The listing builds one solid part. Answer for the finished solid, in the listing's coordinates (mm). Coordinates: 2 decimals unless noted, no trailing zeros. Write each loop counter-clockwise with the first axis right and the second up, starting at its lowest first coordinate (ties: lowest second). Pieces come first, ordered by that corner, then holes. Notation, with made-up numbers: M 10.25,34.25 L 67.25,34.25 A23 ccw 67.25,45.25 Z; hole C 75,-27.75 d2. An arc over 180 degrees is marked long. Answer as a JSON object with one key per item and string values. Group by question number.
from build123d import *

# Parameters (mm, degrees)
SKETCH1_R           = 2.8
BOSS_EXTRUDE1_DEPTH = 4.7625


with BuildPart() as part:
    # Sketch1 → Boss-Extrude1 (new body)
    with BuildSketch(Plane.XY):
        with BuildLine():
            Line((103.944676345, 0), (-249.362453306, 0))
            ThreePointArc((-249.362453306, 0), (-262.056114412, 7.008068585), (-262.888702501, 21.483870968))
            Line((-262.888702501, 21.483870968), (-44.090322581, 477.927471542))
            Line((-44.090322581, 477.927471542), (-26.055323655, 469.282310251))
            Line((-26.055323655, 469.282310251), (103.944676345, 469.282310251))
            ThreePointArc((103.944676345, 469.282310251), (118.086811969, 463.424445875), (123.944676345, 449.282310251))
            Line((123.944676345, 449.282310251), (123.944676345, 20))
            ThreePointArc((123.944676345, 20), (118.086811969, 5.857864376), (103.944676345, 0))
        make_face()
        with Locations((-52.174961355, 437.927471542)):
            Circle(SKETCH1_R, mode=Mode.SUBTRACT)
        with Locations((-142.258875916, 250)):
            Circle(SKETCH1_R, mode=Mode.SUBTRACT)
        with Locations((-242.923360477, 40)):
            Circle(SKETCH1_R, mode=Mode.SUBTRACT)
    extrude(amount=-BOSS_EXTRUDE1_DEPTH)


solid = part.part
Item 1: A cutting plane is placed at C-C, the plane x = -89.5. Write down the section's boundary in (y, z), and give its area (3 significant figures).
Item 2: For a pull along X with two mould halves and no side action, classify faces 1 (the face through (-155.02, 246.51, -2.35)), 2 (the face through (117.93, 463.58, -2.35)), 3 (the face through (-24, 189, -4.762)) as +X half, -X half, draft (parallel to the pull), parting line (faces both ways), or undercut.
Item 3: A flat-ended cylindrical pin translates along its axis: pin 1 Ø5 at (x, y) = (-142.26, 250) entering from +Z. Find the tip coordinate at first contact, or state that the pin passes through.
Item 4: A cutting plane is placed at B-B, the plane y = 264. Write down the section's boundary in (x, z).
Item 5: Consider L1, parallel to X at y = 250, z = -1.85; L2, parallel to Y at x = 34, z = -0.4; L3, parallel to Y at x = -241, z = -1.9. Determine where each line is inside the solid, lowest interval first. Write a range as from..to.
Item 6: A cutting plane is placed at A-A, the plane z = -3. Write down the section's boundary in (x, y), and give its area (3 significant figures).
Answer:
{
 "1": {"outline": "M 0,-4.76 L 383.2,-4.76 L 383.2,0 L 0,0 Z", "area": "1,820 mm2"},
 "2": {"face 1": "-X half", "face 2": "+X half", "face 3": "draft"},
 "3": {"pin 1": "through"},
 "4": {"outline": "M -146.64,-4.76 L 123.94,-4.76 L 123.94,0 L -146.64,0 Z"},
 "5": {"L1": "-153.35..-145.06, -139.46..123.94", "L2": "0..469.28", "L3": "0..37.97, 42.03..67.15"},
 "6": {"outline": "M -262.89,21.48 A15 ccw -249.36,0 L 103.94,0 A20 ccw 123.94,20 L 123.94,449.28 A20 ccw 103.94,469.28 L -26.06,469.28 L -44.09,477.93 Z; hole C -242.92,40 d5.6; hole C -142.26,250 d5.6; hole C -52.17,437.93 d5.6", "area": "133,000 mm2"}
}
